from build123d import *

# Parameters (mm, degrees)
F0_R      = 1
F1_DEPTH  = 5.5
F2_W      = 5.5
F2_H      = 57
F3_DEPTH  = 25
F4_DEPTH  = 5
F6_DEPTH  = 25
F7_W      = 8
F7_H      = 8
F8_DEPTH  = 1.5
F9_R      = 1
F10_DEPTH = 25


with BuildPart() as f1:
    # F0 (on Front) → F1 (new body)
    with BuildSketch(Plane.XZ):
        with BuildLine():
            ThreePointArc((-37.7052051574, 84.6366998268), (-39.9019042985, 89.9400006857), (-45.2052051574, 92.1366998268))
            ThreePointArc((-45.2052051574, 92.1366998268), (-50.5085060163, 89.9400006857), (-52.7052051574, 84.6366998268))
            ThreePointArc((-52.7052051574, 84.6366998268), (-45.2052051574, 77.1366998268), (-37.7052051574, 84.6366998268))
        make_face()
        with Locations((-45.2052051574, 84.6366998268)):
            Circle(F0_R, mode=Mode.SUBTRACT)
        with BuildLine():
            ThreePointArc((-37.7052051574, 84.6366998268), (-45.2052051574, 77.1366998268), (-52.7052051574, 84.6366998268))
            Line((-52.7052051574, 84.6366998268), (-52.7052051574, -7.8633001732))
            Line((-52.7052051574, -7.8633001732), (-37.7052051574, -7.8633001732))
            Line((-37.7052051574, -7.8633001732), (-37.7052051574, 84.6366998268))
        make_face()
    extrude(amount=F1_DEPTH)

    # F2 (on face) → F3 (cut)
    with BuildSketch(Plane(origin=(-52.7052051574, 0, 0), x_dir=(0, -1, 0), z_dir=(-1, 0, 0))):
        with Locations((2.75, 20.6366998268)):
            Rectangle(F2_W, F2_H)
    extrude(amount=-F3_DEPTH, mode=Mode.SUBTRACT)

    # F4 (add): a face of the model
    f4_faces = [f1.faces().sort_by_distance(p)[0] for p in [
        (-52.7052051574, -2.75, 66.8866998268),
    ]]
    extrude(f4_faces, amount=F4_DEPTH)

    # F5 (on face) → F6 (cut)
    with BuildSketch(Plane.XZ.offset(5.5)):
        Polygon((-57.7052051574, 49.1366998268), (-52.7052051574, 84.6366998268), (-57.7052051574, 84.6366998268), align=None)
    extrude(amount=-F6_DEPTH, mode=Mode.SUBTRACT)

    # F7 (on face) → F8 (join)
    with BuildSketch(Plane(origin=(0, 0, 0), x_dir=(-1, 0, 0), z_dir=(0, 1, 0))):
        with Locations((47.7052051574, 53.1366998268)):
            Rectangle(F7_W, F7_H)
    extrude(amount=F8_DEPTH)

    # F9 (on face) → F10 (cut)
    with BuildSketch(Plane(origin=(0, 1.5, 0), x_dir=(-1, 0, 0), z_dir=(0, 1, 0))):
        with Locations((47.7052051574, 53.1366998268)):
            Circle(F9_R)
    extrude(amount=-F10_DEPTH, mode=Mode.SUBTRACT)


solid = f1.part
Here's how the part is built. I have some questions about the finished solid (model axes, mm). A direction names the side the tool comes from. Give positions to 0.01 mm unless a question says otherwise; leave off trailing zeros. Order: outer loops, then holes, each group sorted by start corner. A loop starts at its lowest first (then second) coordinate and runs counter-clockwise, first axis right, second up. Notation, with made-up numbers: (55.25, -31.5) -> (86.25, -31.5) arc R12 cw to (86.25, -8.5) -> close; hole circle Ø4 at (19, -32.5). An arc over 180 degrees is marked (long way). Use a Markdown table: item, result. Add a question column.
Item 1: For faces 5 (the face through (-45, -5.5, 71)), 6 (the face through (-48, 1, 57.137)), 7 (the face through (-51.705, 1, 53)), which set-ups out of +Z, -Z, +X, -X, +Y, -Y let a thin tool reach every point of the face, with its end or its side?
Item 2: Imagine slicing it at A-A on x = -48. Please give me the cut outline in (y, z).
Item 3: Imagine slicing it at D-D on z = 71.5. Please give me the cut outline in (x, y), plus the area to 3 significant figures.
Item 4: If we mould it in two halves opening along X, with no side actions, what happens to faces 1 (the face through (-46.968, -1.951, 53.813)), 2 (the face through (-44.74, -2.71, 83.75)), 3 (the face through (-48, -3, 49.137)), 4 (the face through (-43.705, 1, 53))? For each: pulls with the +X half, pulls with the -X half, needs draft (parallel to the pull), parting line crosses it, or undercut.
Item 5: Will these pins go through, and if not, where does the flat tip stop? pin 1 (1.6 mm diameter, centred on x = -48.5, y = 1, fed in from +Z); pin 2 (1.2 mm diameter, centred on y = 1, z = 52.5, fed in from -X); pin 3 (10 mm diameter, centred on x = -43.5, z = 67.5, fed in from +Y).
Item 6: Imagine slicing it at C-C on x = -44.75. Please give me the cut outline in (y, z).
Item 7: Imagine slicing it at B-B on y = 0.75. Please give me the cut outline in (x, z).
Item 8: I need wall thicknesses on line 1 (Y direction, x = -53, z = 68.5); line 2 (X direction, y = -2.75, z = 54); line 3 (X direction, y = -1.75, z = 85.5). Which ranges of each line are inside material? Lowest first, please.
Data:
| question | item | result |
|---|---|---|
| 1 | face 5 | +Z, -Z, +X, -X, -Y |
| 1 | face 6 | +Z, +X, -X, +Y |
| 1 | face 7 | +Z, -Z, -X, +Y |
| 2 | outline | (-5.5, 49.14) -> (1.5, 49.14) -> (1.5, 52.18) -> (-5.5, 52.18) -> close; (-5.5, 54.09) -> (1.5, 54.09) -> (1.5, 57.14) -> (0, 57.14) -> (0, 91.6) -> (-5.5, 91.6) -> close |
| 3 | outline | (-54.56, -5.5) -> (-37.71, -5.5) -> (-37.71, 0) -> (-54.56, 0) -> close |
| 3 | area | 92.7 mm² |
| 4 | face 1 | undercut |
| 4 | face 2 | undercut |
| 4 | face 3 | needs draft |
| 4 | face 4 | pulls with the +X half |
| 5 | pin 1 | stops at z = 57.14 |
| 5 | pin 2 | stops at x = -51.71 |
| 5 | pin 3 | stops at y = 0 |
| 6 | outline | (-5.5, 49.14) -> (1.5, 49.14) -> (1.5, 57.14) -> (0, 57.14) -> (0, 83.75) -> (-5.5, 83.75) -> close; (-5.5, 85.53) -> (0, 85.53) -> (0, 92.12) -> (-5.5, 92.12) -> close |
| 7 | outline | (-51.71, 49.14) -> (-43.71, 49.14) -> (-43.71, 57.14) -> (-51.71, 57.14) -> close; hole circle Ø2 at (-47.71, 53.14) |
| 8 | line 1 | y = -5.5 to 0 |
| 8 | line 2 | x = -57.02 to -48.21, -47.2 to -37.71 |
| 8 | line 3 | x = -52.66 to -45.71, -44.7 to -37.76 |
